Part print with two shaded views. Sizes in mm from the minimum x, y, z corner. A direction names the side the tool comes from. Round coordinates to 2 decimals unless told otherwise and drop trailing zeros. Order: outer loops, then holes, each group sorted by start corner. A loop starts at its lowest first (then second) coordinate and runs counter-clockwise, first axis right, second up. Notation, with made-up numbers: (-2.75, 51.25) -> (15.25, 51.25) arc R16 ccw to (15.25, 80.25) -> close; hole circle Ø6 at (-4, -20). An arc over 180 degrees is marked (long way). Use a Markdown table: item, result. Add a question column.
Item 1: Slice it at A-A, the plane x = 15. Give the cut face in (y, z), plus the area to 3 significant figures.
Item 2: 3-axis set-ups, long thin cutter, end or side, ignore diameter. For the marked faces 4 and 5: which of +Z, -Z, +X, -X, +Y, -Y reach the whole face in a straight line?
Item 3: Probe L1, parallel to Y at x = 15, z = 13.4; L2, parallel to Z at x = 12, y = 9; L3, parallel to X at y = 15, z = 4. List the from-to ranges inside material, lowest first.
Item 4: Two-plate mould, pull along Y, no slides. Class the marked faces 1, 2 and 3: released by +Y, released by -Y, zero draft, split by the parting line, or undercut.
Item 5: Slice it at B-B, the plane z = 6.5. Give the cut face in (x, y).
Item 6: Slice it at D-D, the plane x = 11.5. Give the cut face in (y, z).
Item 7: Slice it at C-C, the plane x = 2.5. Give the cut face in (y, z).
Item 8: Pin check, flat tips, straight feed: pin 1 (9.5 mm diameter, centred on x = 15, y = 75, fed in from +Z); pin 2 (5 mm diameter, centred on x = 20, z = 11, fed in from -Y); pin 3 (1 mm diameter, centred on y = 80, z = 13, fed in from +X); pin 4 (8 mm diameter, centred on x = 26.5, z = 5.5, fed in from -Y). Stop position of each tip, or through.
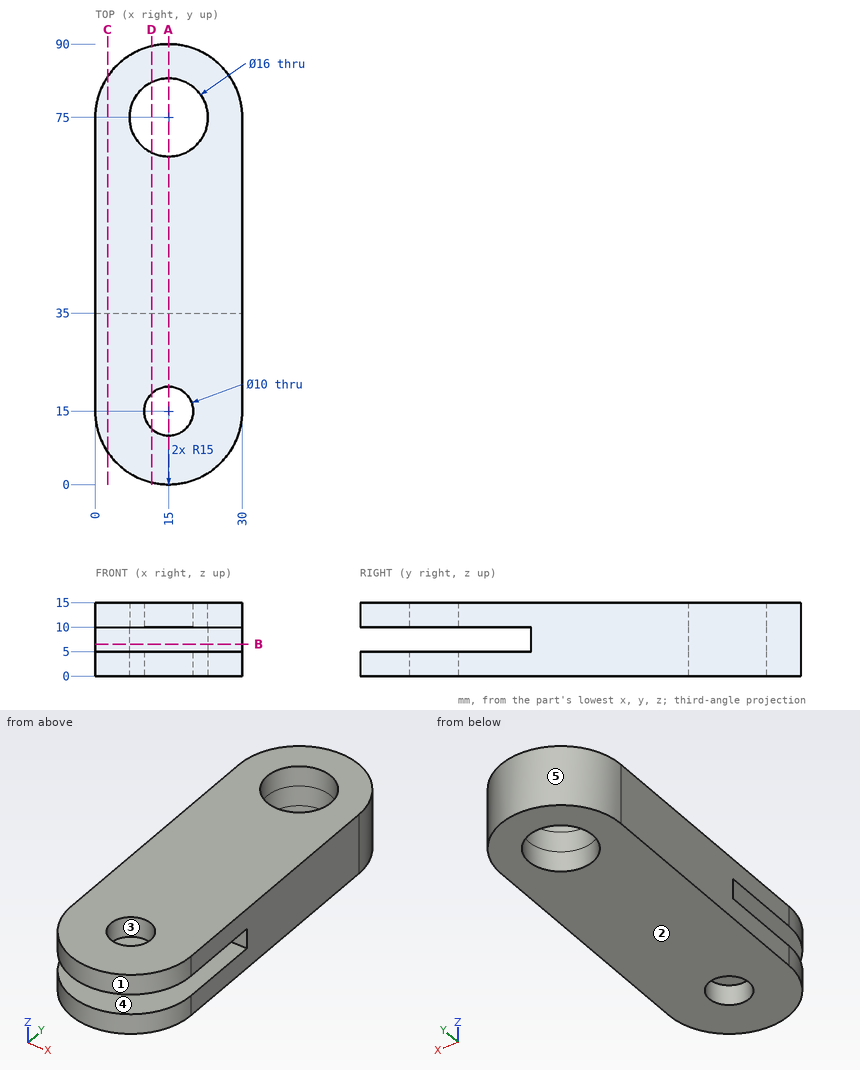
Check sheet entries:
| question | item | result |
|---|---|---|
| 1 | outline | (0, 0) -> (10, 0) -> (10, 5) -> (0, 5) -> close; (0, 10) -> (10, 10) -> (10, 15) -> (0, 15) -> close; (20, 0) -> (67, 0) -> (67, 15) -> (20, 15) -> (20, 10) -> (35, 10) -> (35, 5) -> (20, 5) -> close; (83, 0) -> (90, 0) -> (90, 15) -> (83, 15) -> close |
| 1 | area | 835 mm2 |
| 2 | face 4 | +X, -X, -Y |
| 2 | face 5 | +Z, -Z, +Y |
| 3 | L1 | 0 to 10, 20 to 67, 83 to 90 |
| 3 | L2 | 0 to 5, 10 to 15 |
| 3 | L3 | 0 to 10, 20 to 30 |
| 4 | face 1 | released by -Y |
| 4 | face 2 | zero draft |
| 4 | face 3 | undercut |
| 5 | outline | (0, 35) -> (30, 35) -> (30, 75) arc R15 ccw to (0, 75) -> close; hole circle Ø16 at (15, 75) |
| 6 | outline | (0.41, 0) -> (11.43, 0) -> (11.43, 5) -> (0.41, 5) -> close; (0.41, 10) -> (11.43, 10) -> (11.43, 15) -> (0.41, 15) -> close; (18.57, 0) -> (67.81, 0) -> (67.81, 15) -> (18.57, 15) -> (18.57, 10) -> (35, 10) -> (35, 5) -> (18.57, 5) -> close; (82.19, 0) -> (89.59, 0) -> (89.59, 15) -> (82.19, 15) -> close |
| 7 | outline | (6.71, 0) -> (83.29, 0) -> (83.29, 15) -> (6.71, 15) -> (6.71, 10) -> (35, 10) -> (35, 5) -> (6.71, 5) -> close |
| 8 | pin 1 | through |
| 8 | pin 2 | y = 0.21 |
| 8 | pin 3 | x = 29.31 |
| 8 | pin 4 | y = 2.03 |
